```python
from build123d import *

# Parameters (mm, degrees)
F0_W      = 30.4
F0_H      = 27.4
F1_DEPTH  = 3
F2_W      = 25.9
F2_H      = 25.9
F3_DEPTH  = 1
F4_W      = 3
F4_H      = 41
F5_DEPTH  = 18
F7_DEPTH  = 25
F8_R      = 1.8
F9_DEPTH  = 25
F10_W     = 27.4
F10_H     = 6.8
F11_DEPTH = 3
F12_R     = 1.5
F13_DEPTH = 3.001
F14_W     = 8.9006384343
F14_H     = 16.5555408895
F15_DEPTH = 25
F16_W     = 9.1082898408
F16_H     = 12.178418237
F17_DEPTH = 25
F18_W     = 2
F18_H     = 37.0905021131
F19_DEPTH = 25
F20_W     = 28.4
F20_H     = 34.2
F21_DEPTH = 10
F22_R     = 1.8
F23_DEPTH = 38.7
F24_R     = 3
F25_DEPTH = 25.7
F26_W     = 25.8796279177
F26_H     = 5.8478018075
F27_DEPTH = 1
F28_W     = 61.7600152118
F28_H     = 2
F29_DEPTH = 25


with BuildPart() as f1:
    # F0 (on Front) → F1 (new body)
    with BuildSketch(Plane.XZ):
        Rectangle(F0_W, F0_H)
    extrude(amount=F1_DEPTH)

    # F2 (on face) → F3 (cut)
    with BuildSketch(Plane.XZ.offset(3)):
        with Locations((1.5, 0)):
            Rectangle(F2_W, F2_H)
    extrude(amount=-F3_DEPTH, mode=Mode.SUBTRACT)

    # F4 (on face) → F5 (join)
    with BuildSketch(Plane(origin=(0, 0, 0), x_dir=(-1, 0, 0), z_dir=(0, 1, 0))):
        with Locations((13.7, 0)):
            Rectangle(F4_W, F4_H)
    extrude(amount=-F5_DEPTH)

    # F6 (on face) → F7 (cut)
    with BuildSketch(Plane.YZ.offset(-12.2)):
        with BuildLine():
            Line((-18, 14.5), (-18, -14.5))
            Line((-18, -14.5), (-8, -14.5))
            ThreePointArc((-8, -14.5), (-4.4644660941, -13.0355339059), (-3, -9.5))
            Line((-3, -9.5), (-3, 9.5))
            ThreePointArc((-3, 9.5), (-4.4644660941, 13.0355339059), (-8, 14.5))
            Line((-8, 14.5), (-18, 14.5))
        make_face()
    extrude(amount=-F7_DEPTH, mode=Mode.SUBTRACT)

    # F8 (on face) → F9 (cut)
    with BuildSketch(Plane.YZ.offset(-12.2)):
        with Locations((-14.7, -17.5)):
            Circle(F8_R)
        with Locations((-14.7, 17.5)):
            Circle(F8_R)
    extrude(amount=-F9_DEPTH, mode=Mode.SUBTRACT)

    # F10 (on Front) → F11 (join)
    with BuildSketch(Plane.XZ):
        with Locations((1.5, 17.1)):
            Rectangle(F10_W, F10_H)
    extrude(amount=F11_DEPTH)

    # F12 (on face) → F13 (cut, through all)
    with BuildSketch(Plane.XZ.offset(3)):
        with Locations((6.8696663434, 17)):
            Circle(F12_R)
    extrude(amount=-F13_DEPTH, mode=Mode.SUBTRACT)

    # F14 (on face) → F15 (cut)
    with BuildSketch(Plane.XZ.offset(3)):
        with Locations((-16.6503192171, -17.7777704448)):
            Rectangle(F14_W, F14_H)
    extrude(amount=F15_DEPTH, mode=Mode.SUBTRACT)

    # F16 (on face) → F17 (cut)
    with BuildSketch(Plane.XZ.offset(3)):
        with Locations((-16.7541449204, -19.7892091185)):
            Rectangle(F16_W, F16_H)
    extrude(amount=-F17_DEPTH, mode=Mode.SUBTRACT)

    # F18 (on face) → F19 (cut)
    with BuildSketch(Plane.XZ.offset(3)):
        with Locations((14.2, 1.9547489434)):
            Rectangle(F18_W, F18_H)
    extrude(amount=-F19_DEPTH, mode=Mode.SUBTRACT)

    # F20 (on face) → F21 (join)
    with BuildSketch(Plane(origin=(0, 0, 0), x_dir=(-1, 0, 0), z_dir=(0, 1, 0))):
        with Locations((1, 3.4)):
            Rectangle(F20_W, F20_H)
    extrude(amount=F21_DEPTH)

    # F22 (on face) → F23 (cut)
    with BuildSketch(Plane.YZ.offset(13.2)):
        with Locations((5.3, 0)):
            Circle(F22_R)
    extrude(amount=-F23_DEPTH, mode=Mode.SUBTRACT)

    # F24 (on face) → F25 (cut)
    with BuildSketch(Plane.YZ.offset(13.2)):
        with Locations((5.3, 0)):
            Circle(F24_R)
    extrude(amount=-F25_DEPTH, mode=Mode.SUBTRACT)

    # F26 (on face) → F27 (cut)
    with BuildSketch(Plane.XZ.offset(3)):
        with Locations((1.4898139589, -15.8739009038)):
            Rectangle(F26_W, F26_H)
    extrude(amount=-F27_DEPTH, mode=Mode.SUBTRACT)

    # F28 (on face) → F29 (cut)
    with BuildSketch(Plane.XZ.offset(3)):
        with Locations((15.6800076059, -12.7)):
            Rectangle(F28_W, F28_H)
    extrude(amount=-F29_DEPTH, mode=Mode.SUBTRACT)


solid = f1.part
```
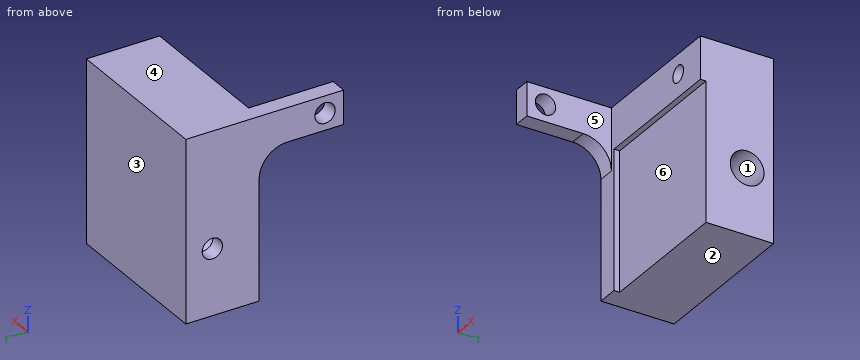
Input: part model. Units: mm. Frame: model coordinates. Face numbers are marked on the shaded views. A direction names the side the tool comes from. Give positions to 0.01 mm unless a question says otherwise; leave off trailing zeros. Loops run counter-clockwise (first coordinate to the right, second up) from the corner with the lowest first, then second, coordinate; pieces in that order, holes last. Notation, with made-up numbers: (-27.5, 34.5) -> (29.5, 34.5) arc R25 ccw to (29.5, 46.5) -> close; hole circle Ø10 at (-8, 52). An arc over 180 degrees is marked (long way). Use a Markdown table: item, result.
Q1. Ray query, probe 1 along Z at (x, y) = (-13.25, 5.3); probe 2 along Z at (x, y) = (-5.25, 5.3); probe 3 along X at (y, z) = (-6, 15.5). Return the intervals inside material, ascending. Write a range as from..to.
Entries:
| item | result |
|---|---|
| probe 1 | z = -11.7..-1.8, 1.8..20.5 |
| probe 2 | z = -11.7..-3, 3..20.5 |
| probe 3 | x = -15.2..-12.2 |
Q2. Section query C-C, the plane x = 4. Return the cut outline in (y, z), plus the area to 3 significant figures.
Entries:
| item | result |
|---|---|
| outline | (-3, 12.95) -> (-2, 12.95) -> (-2, -11.7) -> (10, -11.7) -> (10, 20.5) -> (-3, 20.5) -> close; hole circle Ø6 at (5.3, 0) |
| area | 366 mm² |
Q3. Section query D-D, the plane z = 17.5. Return the cut outline in (x, y), plus the area to 3 significant figures.
Entries:
| item | result |
|---|---|
| outline | (-15.2, -18) -> (-12.2, -18) -> (-12.2, -16.5) -> (-15.2, -16.5) -> close; (-15.2, -12.9) -> (-12.2, -12.9) -> (-12.2, -3) -> (5.46, -3) -> (5.46, 0) -> (8.28, 0) -> (8.28, -3) -> (13.2, -3) -> (13.2, 10) -> (-15.2, 10) -> close |
| area | 395 mm² |
Q4. Section query A-A, the plane y = 5.3. Return the cut outline in (x, z).
Entries:
| item | result |
|---|---|
| outline | (-15.2, -11.7) -> (13.2, -11.7) -> (13.2, -3) -> (-12.5, -3) -> (-12.5, -1.8) -> (-15.2, -1.8) -> close; (-15.2, 1.8) -> (-12.5, 1.8) -> (-12.5, 3) -> (13.2, 3) -> (13.2, 20.5) -> (-15.2, 20.5) -> close |
Q5. Section query B-B, the plane z = 0. Return the cut outline in (x, y).
Entries:
| item | result |
|---|---|
| outline | (-15.2, -3) -> (-11.45, -3) -> (-11.45, -2) -> (13.2, -2) -> (13.2, 2.3) -> (-12.5, 2.3) -> (-12.5, 3.5) -> (-15.2, 3.5) -> close; (-15.2, 7.1) -> (-12.5, 7.1) -> (-12.5, 8.3) -> (13.2, 8.3) -> (13.2, 10) -> (-15.2, 10) -> close |
Q6. Access query for the marked faces 4, 5 and 6. Directions: +Z, -Z, +X, -X, +Y, -Y. A direction counts if a zero-diameter tool reaches every point of the face in a straight line with its end or side. Return the directions, or none.
Entries:
| item | result |
|---|---|
| face 4 | +Z, +X, -X, +Y, -Y |
| face 5 | +Z, -Z, +X, -Y |
| face 6 | -Z, +X, -Y |
Q7. Pull-direction query (Z, two-part tool) for the marked faces 1, 2 and 3; classes: pulls with the +Z half, pulls with the -Z half, needs draft (parallel to the pull), parting line crosses it, or undercut.
Entries:
| item | result |
|---|---|
| face 1 | undercut |
| face 2 | pulls with the -Z half |
| face 3 | needs draft |
Q8. First-contact query: P1, Ø9.5, axis at y = 5.3, z = 0, coming from the +X side; P2, Ø0.5, axis at x = 2, y = -2.5, coming from the -Z side; P3, Ø12, axis at y = -13, z = 14.5, coming from the +X side; P4, Ø0.5, axis at y = -2.5, z = 1.5, coming from the +X side. Flat tips, straight axial feed; report the tip coordinate or a pass-through.
Entries:
| item | result |
|---|---|
| P1 | stops at x = 13.2 |
| P2 | stops at z = 12.95 |
| P3 | stops at x = -12.2 |
| P4 | stops at x = -11.45 |
